CAD build for the part. Positions are in the model's coordinates, mm. Coordinates: 2 decimals unless noted, no trailing zeros. Loops run counter-clockwise (first coordinate to the right, second up) from the corner with the lowest first, then second, coordinate; pieces in that order, holes last. Notation, with made-up numbers: (79.5, 28.5) -> (100.5, 28.5) arc R18 ccw to (100.5, 47.5) -> close; hole circle Ø4 at (-32, 85.25). An arc over 180 degrees is marked (long way). Answer as a JSON object with one key per item and string values. Group by question number.
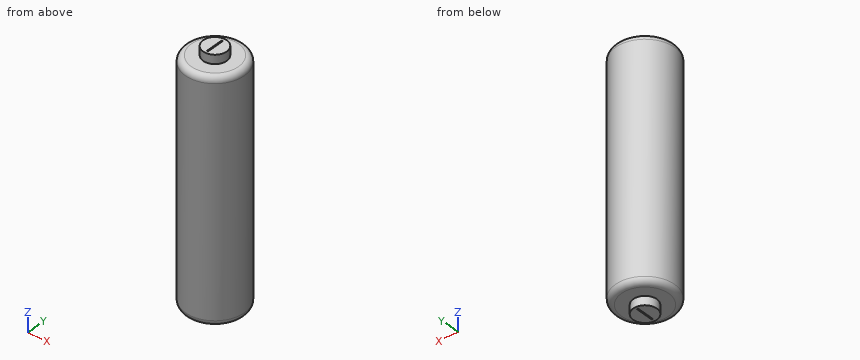
from build123d import *

# Parameters (mm, degrees)
SKETCH1_R           = 250
BOSS_EXTRUDE4_DEPTH = 1000
SKETCH6_R           = 100
BOSS_EXTRUDE5_DEPTH = 75
SKETCH8_W           = 10
SKETCH8_H           = 150
CUT_EXTRUDE7_DEPTH  = 10
FILLET1_R           = 50


with BuildPart() as part:
    # Sketch1 → Boss-Extrude4 (new, symmetric)
    with BuildSketch(Plane.XY):
        Circle(SKETCH1_R)
    extrude(amount=BOSS_EXTRUDE4_DEPTH, both=True)

    # Sketch6 → Boss-Extrude5 (add, symmetric)
    with BuildSketch(Plane.XY.offset(1000)):
        Circle(SKETCH6_R)
    boss_extrude5 = extrude(amount=BOSS_EXTRUDE5_DEPTH, both=True)

    # Sketch8 → Cut-Extrude7 (cut)
    with BuildSketch(Plane.XY.offset(1075)):
        Rectangle(SKETCH8_W, SKETCH8_H)
    cut_extrude7 = extrude(amount=-CUT_EXTRUDE7_DEPTH, mode=Mode.SUBTRACT)

    # Mirror3: Boss-Extrude5, Cut-Extrude7 across plane
    add(boss_extrude5.mirror(Plane.XY))
    add(cut_extrude7.mirror(Plane.XY), mode=Mode.SUBTRACT)

    # Fillet1
    fillet1_edges = [part.edges().sort_by_distance(p)[0] for p in [
        (-250, 0, -1000),
        (-250, 0, 1000),
    ]]
    fillet(fillet1_edges, radius=FILLET1_R)


solid = part.part
Item 1: Flat gauge pins, fed straight in: P1, Ø11, axis at y = 30, z = 1071, coming from the -X side; P2, Ø11, axis at y = -1, z = -1072, coming from the +X side; P3, Ø1, axis at x = -51, y = -182, coming from the +Z side. Where does each tip first touch, or does it go through?
Item 2: Band-saw the part on B-B, the plane z = -677.5. List the corners of the cut face in (x, y), and give its area (3 significant figures).
Item 3: Drill centre lines: L1, parallel to Z at x = -76, y = -188.5; L2, parallel to Z at x = -73, y = 191; L3, parallel to Y at x = -52.5, z = 643.5. Where is each one in solid material? Low to high.
Item 4: Band-saw the part on A-A, the plane y = 0. List the corners of the cut face in (x, z).
Reply:
{
 "1": {"P1": "x = -96.95", "P2": "x = 100", "P3": "z = 1000"},
 "2": {"outline": "circle Ø500 at (0, 0)", "area": "196,000 mm²"},
 "3": {"L1": "-999.89 to 999.89", "L2": "-999.8 to 999.8", "L3": "-244.43 to 244.43"},
 "4": {"outline": "(-250, -950) arc R50 ccw to (-200, -1000) -> (-100, -1000) -> (-100, -1075) -> (-5, -1075) -> (-5, -1065) -> (5, -1065) -> (5, -1075) -> (100, -1075) -> (100, -1000) -> (200, -1000) arc R50 ccw to (250, -950) -> (250, 950) arc R50 ccw to (200, 1000) -> (100, 1000) -> (100, 1075) -> (5, 1075) -> (5, 1065) -> (-5, 1065) -> (-5, 1075) -> (-100, 1075) -> (-100, 1000) -> (-200, 1000) arc R50 ccw to (-250, 950) -> close"}
}
